Could you check a few things on this model? Use its own coordinates, in mm. A direction names the side the tool comes from. Give positions to 0.01 mm unless a question says otherwise; leave off trailing zeros. Loops run counter-clockwise (first coordinate to the right, second up) from the corner with the lowest first, then second, coordinate; pieces in that order, holes last. Notation, with made-up numbers: M 10.25,11 L 26.25,11 A13 cw 26.25,26 Z; hole C -37.75,-17 d5. An arc over 180 degrees is marked long. Return JSON: item names as keys, results as strings. Group by question number.
1. Please list where these lines run through material, in increasing order: line 1 (Y direction, x = 0, z = 2); line 2 (Z direction, x = -7.75, y = -6); line 3 (Z direction, x = 2.25, y = 0).
2. If we section it at B-B (z = 11.5): Write out the boundary of the cut face in (x, y).
3. For faces 4 (the flat face through (-3.25, 0, 10)), 5 (the cylindrical face through (-1.43, -2.75, 3.45)), 6 (the cylindrical face through (-2.17, -9.76, 0.74)), which set-ups out of +Z, -Z, +X, -X, +Y, -Y let a thin tool reach every point of the face, with its end or its side?
4. If we section it at A-A (x = 0): Write out the boundary of the cut face in (y, z).
5. If we mould it in two halves opening along X, with no side actions, what happens to faces 1 (the flat face through (2, 7, 1.5)), 2 (the flat face through (0, 9, 0.75)), 3 (the flat face through (3.25, 0, 10))? For each: +X half, -X half, draft (parallel to the pull), parting line (faces both ways), or undercut.
6. For pin 1 (1.8 mm diameter, centred on y = 0, z = 10, fed in from +X); pin 2 (8 mm diameter, centred on x = -6.5, z = 8.5, fed in from +Y); pin 3 (3 mm diameter, centred on y = 6, z = 6, fed in from -X); pin 4 (2 mm diameter, centred on x = 6, z = 7.5, fed in from +Y), each with a flat end and sliding along its axis, tell me the tip position at first contact or that it passes through.
```python
from build123d import *

# Parameters (mm, degrees)
SKETCH1_R           = 10
BOSS_EXTRUDE1_DEPTH = 1.5
BOSS_EXTRUDE2_DEPTH = 12.5
CUT_EXTRUDE2_START  = -0.75
CUT_EXTRUDE2_DEPTH  = 0.75
SKETCH5_R           = 3.1
CUT_EXTRUDE3_DEPTH  = 7
FILLET5_SIZE        = 3.75
FILLET5_SIZE_2      = 6
FILLET6_R           = 0.5


with BuildPart() as part:
    # Sketch1 → Boss-Extrude1 (new body)
    with BuildSketch(Plane.XY):
        Circle(SKETCH1_R)
    extrude(amount=BOSS_EXTRUDE1_DEPTH)

    # Sketch2 → Boss-Extrude2 (add)
    with BuildSketch(Plane.XY.offset(1.5)):
        with BuildLine():
            Line((-3.25, 6.199798384), (-3.25, -6.199798384))
            ThreePointArc((-3.25, -6.199798384), (0, -7), (3.25, -6.199798384))
            Line((3.25, -6.199798384), (3.25, 6.199798384))
            ThreePointArc((3.25, 6.199798384), (0, 7), (-3.25, 6.199798384))
        make_face()
    extrude(amount=BOSS_EXTRUDE2_DEPTH)

    # Sketch4 → Cut-Extrude2 (cut)
    with BuildSketch(Plane.XY.offset(1.5).offset(CUT_EXTRUDE2_START)):
        with BuildLine():
            Line((-0.5, 9.987492178), (-0.5, 7.987492178))
            Line((-0.5, 7.987492178), (0.5, 7.987492178))
            Line((0.5, 7.987492178), (0.5, 9.987492178))
            ThreePointArc((0.5, 9.987492178), (0, 10), (-0.5, 9.987492178))
        make_face()
    extrude(amount=CUT_EXTRUDE2_DEPTH, mode=Mode.SUBTRACT)

    # Sketch5 → Cut-Extrude3 (cut)
    with BuildSketch(Plane(origin=(0, 0, 0), x_dir=(-1, 0, 0), z_dir=(0, 0, -1))):
        Circle(SKETCH5_R)
    extrude(amount=-CUT_EXTRUDE3_DEPTH, mode=Mode.SUBTRACT)

    # Fillet5
    # a fillet whose section is not a circle: 6, 3.75 mm, written as the material it adds along each edge
    with BuildSketch(Plane(origin=(-3.25, 21.199798384, 1.5), x_dir=(-1, 0, 0), z_dir=(0, -1, 0))) as fillet5_piece_1_section:
        with BuildLine():
            Bezier((FILLET5_SIZE, 0), (0, 0), (0, -FILLET5_SIZE_2), weights=[1, 0.333333333, 1])
            Line((0, -FILLET5_SIZE_2), (0, 0))
            Line((0, 0), (FILLET5_SIZE, 0))
        make_face()
    fillet5_piece_1 = extrude(amount=42.399596768, mode=Mode.PRIVATE)
    fillet5_piece_1 = fillet5_piece_1 & Plane(origin=(0, 0, 1.5), x_dir=(0.4642857142857146, 0.8856854834026602, 0), z_dir=(0, 0, -1)) * Cylinder(7, 109, mode=Mode.PRIVATE)
    add(fillet5_piece_1)
    with BuildSketch(Plane(origin=(3.25, -21.199798384, 1.5), x_dir=(1, 0, 0), z_dir=(0, 1, 0))) as fillet5_piece_2_section:
        with BuildLine():
            Bezier((FILLET5_SIZE, 0), (0, 0), (0, -FILLET5_SIZE_2), weights=[1, 0.333333333, 1])
            Line((0, -FILLET5_SIZE_2), (0, 0))
            Line((0, 0), (FILLET5_SIZE, 0))
        make_face()
    fillet5_piece_2 = extrude(amount=42.399596768, mode=Mode.PRIVATE)
    fillet5_piece_2 = fillet5_piece_2 & Plane(origin=(0, 0, 1.5), x_dir=(0.4642857142857146, 0.8856854834026602, 0), z_dir=(0, 0, -1)) * Cylinder(7, 109, mode=Mode.PRIVATE)
    add(fillet5_piece_2)

    # Fillet6
    fillet6_edges = [part.edges().sort_by_distance(p)[0] for p in [
        (3.25, 0, 14),
        (0, -7, 14),
        (-3.25, 0, 14),
        (0, 7, 14),
    ]]
    fillet(fillet6_edges, radius=FILLET6_R)


solid = part.part
```
Answer:
{
 "1": {"line 1": "y = -7 to -3.1, 3.1 to 7", "line 2": "z = 0 to 1.5", "line 3": "z = 7 to 14"},
 "2": {"outline": "M -3.25,-6.2 A7 ccw 3.25,-6.2 L 3.25,6.2 A7 ccw -3.25,6.2 Z"},
 "3": {"face 4": "+Z, -X, +Y, -Y", "face 5": "-Z", "face 6": "+Z, -Z"},
 "4": {"outline": "M -10,0 L -3.1,0 L -3.1,7 L 3.1,7 L 3.1,0 L 10,0 L 10,0.75 L 7.99,0.75 L 7.99,1.5 L 7,1.5 L 7,13.5 A0.5 ccw 6.5,14 L -6.5,14 A0.5 ccw -7,13.5 L -7,1.5 L -10,1.5 Z"},
 "5": {"face 1": "draft", "face 2": "undercut", "face 3": "+X half"},
 "6": {"pin 1": "stops at x = 3.25", "pin 2": "stops at y = 6.54", "pin 3": "stops at x = -4.2", "pin 4": "passes through"}
}
